```python
from build123d import *

# Parameters (mm, degrees)
BOSS_EXTRU_1_DEPTH      = 7
ESQUISSE3_R             = 1.5
ENL_V_MAT_EXTRU_2_DEPTH = 8.5
ESQUISSE4_R             = 2
ENL_V_MAT_EXTRU_3_DEPTH = 19.391574158
ENL_V_MAT_EXTRU_4_DEPTH = 18.727097901


with BuildPart() as part:
    # Esquisse1 → Boss.-Extru.1 (new, symmetric)
    with BuildSketch(Plane.XY):
        with BuildLine():
            Line((-15.5, 0), (-6.25, 0))
            Line((-6.25, 0), (-6.25, 2.5))
            ThreePointArc((-6.25, 2.5), (-6.118164456, 3.776935273), (-5.728219619, 5))
            Line((-5.728219619, 5), (5.728219619, 5))
            ThreePointArc((5.728219619, 5), (6.118164456, 3.776935273), (6.25, 2.5))
            Line((6.25, 2.5), (6.25, 0))
            Line((6.25, 0), (15.5, 0))
            Line((15.5, 0), (15.5, 2))
            Line((15.5, 2), (8.75, 2))
            Line((8.75, 2), (8.75, 7))
            Line((8.75, 7), (-8.75, 7))
            Line((-8.75, 7), (-8.75, 2))
            Line((-8.75, 2), (-15.5, 2))
            Line((-15.5, 2), (-15.5, 0))
        make_face()
    extrude(amount=BOSS_EXTRU_1_DEPTH, both=True)

    # Esquisse3 → Enlèv. mat.-Extru.2 (cut)
    with BuildSketch(Plane(origin=(0, 2, 0), x_dir=(1, 0, 0), z_dir=(0, 1, 0))):
        with Locations(Location((-12.125, 0, 0), (0, 0, 180))):
            Circle(ESQUISSE3_R)
        with Locations(Location((12.125, 0, 0), (0, 0, 270))):
            Circle(ESQUISSE3_R)
    extrude(amount=-ENL_V_MAT_EXTRU_2_DEPTH, mode=Mode.SUBTRACT)

    # Esquisse4 → Enlèv. mat.-Extru.3 (cut, through all)
    with BuildSketch(Plane(origin=(0, 7, 0), x_dir=(1, 0, 0), z_dir=(0, 1, 0))):
        with Locations(Location((0, 0, 0), (0, 0, 270))):
            Circle(ESQUISSE4_R)
    extrude(amount=-ENL_V_MAT_EXTRU_3_DEPTH, mode=Mode.SUBTRACT)

    # Esquisse5 → Enlèv. mat.-Extru.4 (cut, through all)
    with BuildSketch(Plane(origin=(0, 2, 0), x_dir=(1, 0, 0), z_dir=(0, 1, 0))):
        with BuildLine():
            add(Edge.make_bspline(
                [(-8.75, 7), (-15.499999991, 4.474226807), (-15.5, 9e-09)],
                knots=[2.170643252, 2.170643252, 2.170643252, 3.141592653, 3.141592653, 3.141592653], degree=2, weights=[1, 0.88445354, 1]))
            Line((-8.75, 7), (-15.5, 7))
            Line((-15.5, 7), (-15.5, 9e-09))
        make_face()
        with BuildLine():
            Line((15.5, 7), (8.75, 7))
            add(Edge.make_bspline(
                [(15.5, 0), (15.5, 4.474226804), (8.75, 7)],
                knots=[0, 0, 0, 0.970949401, 0.970949401, 0.970949401], degree=2, weights=[1, 0.88445354, 1]))
            Line((15.5, 0), (15.5, 7))
        make_face()
        with BuildLine():
            add(Edge.make_bspline(
                [(-15.5, 9e-09), (-15.500000009, -4.474226801), (-8.75, -7)],
                knots=[3.141592653, 3.141592653, 3.141592653, 4.112542055, 4.112542055, 4.112542055], degree=2, weights=[1, 0.88445354, 1]))
            Line((-15.5, 9e-09), (-15.5, -7))
            Line((-15.5, -7), (-8.75, -7))
        make_face()
        with BuildLine():
            Line((15.5, -7), (15.5, 0))
            add(Edge.make_bspline(
                [(8.75, -7), (15.5, -4.474226804), (15.5, 0)],
                knots=[5.312235906, 5.312235906, 5.312235906, 6.283185307, 6.283185307, 6.283185307], degree=2, weights=[1, 0.88445354, 1]))
            Line((8.75, -7), (15.5, -7))
        make_face()
    extrude(amount=-ENL_V_MAT_EXTRU_4_DEPTH, mode=Mode.SUBTRACT)


solid = part.part
```
Geometry check sheet. Reference: the model listing, model coordinates, mm. A direction names the side the tool comes from. Coordinates: 2 decimals unless noted, no trailing zeros. Order: outer loops, then holes, each group sorted by start corner. A loop starts at its lowest first (then second) coordinate and runs counter-clockwise, first axis right, second up. Notation, with made-up numbers: (-31, 61.5) - (9, 61.5) arc R30 ccw to (9, 85.5) - close; hole circle Ø7 at (-11.75, 70). An arc over 180 degrees is marked (long way). Answer as a JSON object with one key per item and string values. Group by question number.
Item 1: Sectioned sample at D-D, the plane z = 1. Give the number of separate pieces and of enclosed holes in the cut face, and give its area (3 significant figures).
Item 2: Draft check along X on faces 1 (the face through (12.58, 1.01, 1.43)), 2 (the face through (0, 6, -7)), 3 (the face through (-8.75, 5, 0)). Enter one of: +X half, -X half, draft (parallel to the pull), parting line (faces both ways), or undercut.
Item 3: Depth check by flat-ended pin: pin 1 Ø1.2 at (y, z) = (1, -1) entering from +X; pin 2 Ø3.5 at (x, z) = (2.5, 2) entering from -Y; pin 3 Ø4 at (y, z) = (4.5, -4) entering from +X; pin 4 Ø8 at (x, z) = (-6.5, 1) entering from -Y. Enter the tip coordinate at first touch or a pass-through.
Item 4: Scan lines: probe 1 along X at (y, z) = (0.5, 1.25); probe 2 along X at (y, z) = (5.9, 0); probe 3 along X at (y, z) = (0.75, -0.75). Record each from-to range of solid material in increasing order.
Item 5: Sectioned sample at B-B, the plane y = 4.25. Record the cut outline in (x, z).
Item 6: Tool access check on faces 4 (the face through (0, 6, 7)), 5 (the face through (8.75, 4, 0)), 6 (the face through (-11.3, 2, -1.5)), 7 (the face through (6.25, 1, 0)). Record the directions out of +Z, -Z, +X, -X, +Y, -Y that give a thin tool (end or side, any length) a straight path to the whole face; none if there is none.
Item 7: Sectioned sample at C-C, the plane y = 6. Record the cut outline in (x, z), and give its area (3 significant figures).
Item 8: Sectioned sample at A-A, the plane x = 0. Record the cut outline in (y, z).
Resolved:
{
 "1": {"separate pieces": "4", "enclosed holes": "0", "area": "71.5 mm^2"},
 "2": {"face 1": "undercut", "face 2": "draft", "face 3": "-X half"},
 "3": {"pin 1": "x = 15.48", "pin 2": "y = 5", "pin 3": "x = 8.75", "pin 4": "y = 0"},
 "4": {"probe 1": "-15.33 to -12.95, -11.3 to -6.25, 6.25 to 11.3, 12.95 to 15.33", "probe 2": "-8.75 to -2, 2 to 8.75", "probe 3": "-15.44 to -13.42, -10.83 to -6.25, 6.25 to 10.83, 13.42 to 15.44"},
 "5": {"outline": "(-8.75, -7) - (-6, -7) - (-6, 7) - (-8.75, 7) - close; (6, -7) - (8.75, -7) - (8.75, 7) - (6, 7) - close"},
 "6": {"face 4": "+Z, +X, -X, +Y, -Y", "face 5": "+Z, -Z, +X, +Y", "face 6": "+Z, -Z, -X, +Y", "face 7": "+Z, -Z, -Y"},
 "7": {"outline": "(-8.75, -7) - (8.75, -7) - (8.75, 7) - (-8.75, 7) - close; hole circle Ø4 at (0, 0)", "area": "232 mm^2"},
 "8": {"outline": "(5, -7) - (7, -7) - (7, -2) - (5, -2) - close; (5, 2) - (7, 2) - (7, 7) - (5, 7) - close"}
}
